from build123d import *

# Parameters (mm, degrees)
SKETCH1_R           = 6.9469
SKETCH1_R_2         = 3.175
BOSS_EXTRUDE1_DEPTH = 1.016
SKETCH2_R           = 6.35
SKETCH2_R_2         = 3.175
BOSS_EXTRUDE2_DEPTH = 3.683


with BuildPart() as part:
    # Sketch1 → Boss-Extrude1 (new body)
    with BuildSketch(Plane.XY):
        Circle(SKETCH1_R)
        Circle(SKETCH1_R_2, mode=Mode.SUBTRACT)
    extrude(amount=BOSS_EXTRUDE1_DEPTH)

    # Sketch2 → Boss-Extrude2 (add)
    with BuildSketch(Plane.XY.offset(1.016)):
        Circle(SKETCH2_R)
        Circle(SKETCH2_R_2, mode=Mode.SUBTRACT)
    extrude(amount=BOSS_EXTRUDE2_DEPTH)

    # Sketch7 → Cut-Revolve2 (revolve, cut)
    with BuildSketch(Plane(origin=(0, 0, 0), x_dir=(0, 0, -1), z_dir=(1, 0, 0))):
        with BuildLine():
            Line((-4.699, 5.207), (-4.699, 3.937))
            ThreePointArc((-4.699, 3.937), (-4.064, 4.572), (-4.699, 5.207))
        make_face()
        with BuildLine():
            Line((0, 5.207), (0, 3.937))
            ThreePointArc((0, 3.937), (-0.635, 4.572), (0, 5.207))
        make_face()
    revolve(axis=Axis((0, 0, 4.699), (0, 0, -1)), mode=Mode.SUBTRACT)


solid = part.part
Part model, mm, in its own coordinate system. A direction names the side the tool comes from. Give positions to 0.01 mm unless a question says otherwise; leave off trailing zeros. Write each loop counter-clockwise with the first axis right and the second up, starting at its lowest first coordinate (ties: lowest second). Pieces come first, ordered by that corner, then holes.
1) Pin check, flat tips, straight feed: pin 1 (1 mm diameter, centred on y = -3.5, z = 1, fed in from +X); pin 2 (1 mm diameter, centred on x = -0.5, z = 3, fed in from -Y). Stop position of each tip, or through.
Resolved:
pin 1: stops at x = 6.27
pin 2: stops at y = -6.35
2) Cut at D-D on y = 5.75. Write the cut outline in (x, z), then the cut area to 3 significant figures.
Resolved:
outline: (-3.9, 0) - (3.9, 0) - (3.9, 1.02) - (2.69, 1.02) - (2.69, 4.7) - (-2.69, 4.7) - (-2.69, 1.02) - (-3.9, 1.02) - close
area: 27.8 mm2
3) Two-plate mould, pull along X, no slides. Class faces 3 (the face through (-1.38, -6.2, 2.83)), 4 (the face through (-3, 2, 4.699)), 5 (the face through (-0.69, -3.1, 2.32)): released by +X, released by -X, zero draft, split by the parting line, or undercut.
Resolved:
face 3: split by the parting line
face 4: zero draft
face 5: undercut
4) Cut at A-A on y = 0. Write the cut outline in (x, z) (3 decimals), then the cut area to 3 significant figures.
Resolved:
outline: (-6.947, 0) - (-5.207, 0) arc R0.635 cw to (-3.937, 0) - (-3.175, 0) - (-3.175, 4.699) - (-3.937, 4.699) arc R0.635 cw to (-5.207, 4.699) - (-6.35, 4.699) - (-6.35, 1.016) - (-6.947, 1.016) - close; (3.175, 0) - (3.937, 0) arc R0.635 cw to (5.207, 0) - (6.947, 0) - (6.947, 1.016) - (6.35, 1.016) - (6.35, 4.699) - (5.207, 4.699) arc R0.635 cw to (3.937, 4.699) - (3.175, 4.699) - close
area: 28.5 mm2
5) Which spindle directions (+Z, -Z, +X, -X, +Y, -Y) get a long thin tool onto all of the face, cutting with end or side? Do faces 1 (the face through (3, -6, 1.016)), 2 (the face through (-5, 2, 4.699)). Say none if no direction does.
Resolved:
face 1: +Z
face 2: +Z, +X, -X, +Y, -Y
6) Probe L1, parallel to X at y = 1.5, z = 4.15; L2, parallel to Y at x = 0, z = 1.1 (3 decimals); L3, parallel to Y at x = -1.75, z = 4.3. List the from-to ranges inside material, lowest first.
Resolved:
L1: x = -6.17 to -4.66, -3.98 to -2.8, 2.8 to 3.98, 4.66 to 6.17
L2: y = -6.35 to -3.175, 3.175 to 6.35
L3: y = -6.1 to -4.75, -3.68 to -2.65, 2.65 to 3.68, 4.75 to 6.1
7) Cut at C-C on z = 1.5. Write the cut outline in (x, y) (3 decimals), then the cut area to 3 significant figures.
Resolved:
outline: circle Ø12.7 at (0, 0); hole circle Ø6.35 at (0, 0)
area: 95.0 mm2
